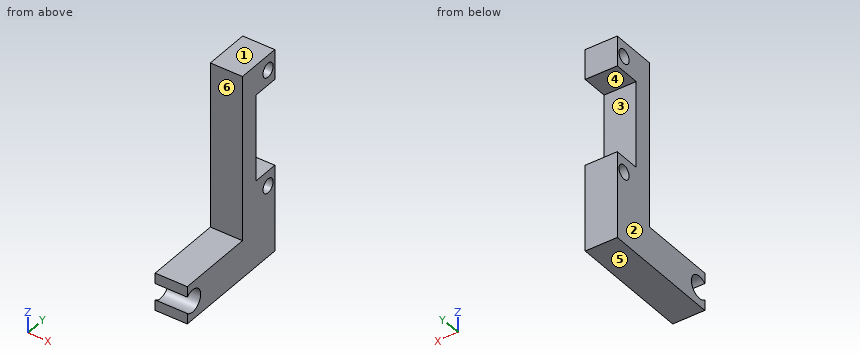
Autodesk Inventor part; units mm, degrees
ref_plane "YZ Plane" through (0, 0, 0) normal (1, 0, 0) x (0, 1, 0)
ref_plane "XZ Plane" through (0, 0, 0) normal (0, 1, 0) x (-1, 0, 0)
ref_plane "XY Plane" through (0, 0, 0) normal (0, 0, 1) x (1, 0, 0)
sketch "Sketch1" plane through (0, 0, 0) normal (1, 0, 0) x (0, 1, 0)
  line L0 (0, 0) -> (0, -8)
  line L1 (0, -8) -> (-7, -8)
  line L2 (-7, -8) -> (-7, -31)
  line L3 (-7, -31) -> (0, -31)
  line L4 (-12, 0) -> (0, 0)
  line L5 (0, -4) -> (-2.5, -4) construction
  circle A0 centre (-2.5, -4) radius 1.875
  line L6 (0, -31) -> (-2.5, -31) construction
  line L7 (-2.5, -31) -> (-2.5, -35) construction
  circle A1 centre (-2.5, -35) radius 1.875
  line L8 (-30.5, -54) -> (0, -54)
  arc A2 (-32.5, -51.1957) -> (-32.5, -46.8043) centre (-30.5, -49) ccw
  line L9 (-30.5, -44) -> (-32.5, -44)
  line L10 (-32.5, -44) -> (-32.5, -46.8043)
  line L11 (-30.5, -54) -> (-32.5, -54)
  line L12 (-32.5, -54) -> (-32.5, -51.1957)
  line L13 (-12, -44) -> (-30.5, -44)
  line L14 (0, -31) -> (0, -54)
  line L15 (-12, 0) -> (-12, -44)
  dimension "d0" = 8
  dimension "d1" = 7
  dimension "d2" = 23
  dimension "d5" = 2.5
  dimension "d6" = 3.75
  dimension "d7" = 4
  dimension "d8" = 3.75
  dimension "d10" = 30.5
  dimension "d11" = 10
  dimension "d13" = 2
extrude "Extrusion1" add sketch "Sketch1" along normal blind 8.5
properties part number "Laser_Holder_1"
Design review of the part built by this model. Coordinates are the model's own, in mm. Face numbers are marked on the shaded views. A direction names the side the tool comes from. Coordinates: 2 decimals unless noted, no trailing zeros. Order: outer loops, then holes, each group sorted by start corner. A loop starts at its lowest first (then second) coordinate and runs counter-clockwise, first axis right, second up. Notation, with made-up numbers: M 41,53.5 L 91,53.5 A29 ccw 91,82.5 Z; hole C 1.25,54.25 d9. An arc over 180 degrees is marked long. Use a Markdown table: item, result.
(1) Wall thickness on probe 1 along Z at (x, y) = (0.75, -2.5) (3 decimals); probe 2 along Z at (x, y) = (3, -30.5); probe 3 along Z at (x, y) = (1, -3): over which ranges is each line inside the solid? List them lowest first.
Worked answers:
| item | result |
|---|---|
| probe 1 | z = -54 to -36.875, -33.125 to -31, -8 to -5.875, -2.125 to 0 |
| probe 2 | z = -54 to -51.97, -46.03 to -44 |
| probe 3 | z = -54 to -36.81, -33.19 to -31, -8 to -5.81, -2.19 to 0 |
(2) Add section B-B (y = -2.5). Give the boundary of the cut face in (x, z) (3 decimals), then the cut area to 3 significant figures.
Worked answers:
| item | result |
|---|---|
| outline | M 0,-54 L 8.5,-54 L 8.5,-36.875 L 0,-36.875 Z; M 0,-33.125 L 8.5,-33.125 L 8.5,-31 L 0,-31 Z; M 0,-8 L 8.5,-8 L 8.5,-5.875 L 0,-5.875 Z; M 0,-2.125 L 8.5,-2.125 L 8.5,0 L 0,0 Z |
| area | 200 mm2 |
(3) Draft analysis for pull direction Z (two halves, no side actions). For the marked faces 1, 2, 3 and 4, state which applies: released by +Z, released by -Z, zero draft, split by the parting line, or undercut.
Worked answers:
| item | result |
|---|---|
| face 1 | released by +Z |
| face 2 | zero draft |
| face 3 | undercut |
| face 4 | undercut |
(4) Add section A-A (y = -30.5). Give the boundary of the cut face in (x, z).
Worked answers:
| item | result |
|---|---|
| outline | M 0,-54 L 8.5,-54 L 8.5,-51.97 L 0,-51.97 Z; M 0,-46.03 L 8.5,-46.03 L 8.5,-44 L 0,-44 Z |
(5) Add section D-D (x = 5). Give the boundary of the cut face in (y, z) (3 decimals).
Worked answers:
| item | result |
|---|---|
| outline | M -32.5,-54 L 0,-54 L 0,-31 L -7,-31 L -7,-8 L 0,-8 L 0,0 L -12,0 L -12,-44 L -32.5,-44 L -32.5,-46.804 A2.97 cw long -32.5,-51.196 Z; hole C -2.5,-35 d3.75; hole C -2.5,-4 d3.75 |
(6) For the marked faces 5 and 6, list the 3-axis set-ups (+Z, -Z, +X, -X, +Y, -Y) from which the entire face can be reached by the end or side of a thin tool; tool diameter is ignored.
Worked answers:
| item | result |
|---|---|
| face 5 | -Z, +X, -X, +Y, -Y |
| face 6 | +Z, +X, -X, -Y |
(7) Add section C-C (z = -35). Give the boundary of the cut face in (x, y) (3 decimals), then the cut area to 3 significant figures.
Worked answers:
| item | result |
|---|---|
| outline | M 0,-12 L 8.5,-12 L 8.5,-4.375 L 0,-4.375 Z; M 0,-0.625 L 8.5,-0.625 L 8.5,0 L 0,0 Z |
| area | 70.1 mm2 |
(8) For P1, Ø3, axis at x = 4, y = -29, coming from the +Z side; P2, Ø4, axis at x = 4.5, z = -11.5, coming from the -Y side; P3, Ø2, axis at y = -2.5, z = -4, coming from the +X side, all flat-tipped, find the tip position at first contact; note any pin that passes through.
Worked answers:
| item | result |
|---|---|
| P1 | stops at z = -44 |
| P2 | stops at y = -12 |
| P3 | passes through |
